from build123d import *

# Parameters (mm, degrees)
F1_DEPTH  = 5
F2_W      = 18
F2_H      = 15
F2_H_2    = 20
F3_DEPTH  = 20
F4_R      = 4
F5_DEPTH  = 25
F6_R      = 1.75
F6_R_2    = 11.25
F7_DEPTH  = 25
F8_W      = 42
F8_H      = 5
F9_DEPTH  = 20
F10_R     = 2.25
F11_DEPTH = 25
F12_DEPTH = 2
F13_R     = 4
F14_R     = 0.6


with BuildPart() as f1:
    # F0 (on Front) → F1 (new body)
    with BuildSketch(Plane.XZ):
        Polygon((-49.7673791122, 6.8827710084), (-49.7673791122, -8.1172289916), (28.2326208878, -8.1172289916), (28.2326208878, 11.8827710084), (10.2326208878, 11.8827710084), (10.2326208878, 46.8827710084), (-31.7673791122, 46.8827710084), (-31.7673791122, 6.8827710084), align=None)
    extrude(amount=F1_DEPTH)

    # F2 (on face) → F3 (join)
    with BuildSketch(Plane.XZ.offset(5)):
        with Locations((-40.7673791122, -0.6172289916)):
            Rectangle(F2_W, F2_H)
        with Locations((19.2326208878, 1.8827710084)):
            Rectangle(F2_W, F2_H_2)
    extrude(amount=F3_DEPTH)

    # F4 (on face) → F5 (cut)
    with BuildSketch(Plane(origin=(0, 0, -8.1172289916), x_dir=(1, 0, 0), z_dir=(0, 0, -1))):
        with Locations((-40.7673791122, 14)):
            Circle(F4_R)
        with Locations((19.2326208878, 14)):
            Circle(F4_R)
    extrude(amount=-F5_DEPTH, mode=Mode.SUBTRACT)

    # F6 (on face) → F7 (cut)
    with BuildSketch(Plane.XZ.offset(5)):
        with Locations((-26.2673791122, 41.3827710084)):
            Circle(F6_R)
        with Locations((-26.2673791122, 10.3827710084)):
            Circle(F6_R)
        with Locations((-10.7673791122, 25.8827710084)):
            Circle(F6_R_2)
        with Locations((4.7326208878, 41.3827710084)):
            Circle(F6_R)
        with Locations((4.7326208878, 10.3827710084)):
            Circle(F6_R)
    extrude(amount=-F7_DEPTH, mode=Mode.SUBTRACT)

    # F8 (on face) → F9 (join)
    with BuildSketch(Plane.XZ.offset(5)):
        with Locations((-10.7673791122, -5.6172289916)):
            Rectangle(F8_W, F8_H)
    extrude(amount=F9_DEPTH)

    # F10 (on face) → F11 (cut)
    with BuildSketch(Plane.XY.offset(-3.1172289916)):
        with Locations((-23.2673791122, -14)):
            Circle(F10_R)
        with Locations((1.7326208878, -14)):
            Circle(F10_R)
    extrude(amount=-F11_DEPTH, mode=Mode.SUBTRACT)

    # F10 (on face) → F12 (cut)
    with BuildSketch(Plane.XY.offset(-3.1172289916)):
        Polygon((-21.24665317, -17.5), (-19.2259272279, -14), (-21.24665317, -10.5), (-25.2881050544, -10.5), (-27.3088309965, -14), (-25.2881050544, -17.5), align=None)
        with Locations((-23.2673791122, -14)):
            Circle(F10_R, mode=Mode.SUBTRACT)
        Polygon((3.75334683, -17.5), (5.7740727721, -14), (3.75334683, -10.5), (-0.2881050544, -10.5), (-2.3088309965, -14), (-0.2881050544, -17.5), align=None)
        with Locations((1.7326208878, -14)):
            Circle(F10_R, mode=Mode.SUBTRACT)
    extrude(amount=-F12_DEPTH, mode=Mode.SUBTRACT)

    # F13
    f13_edges = [f1.edges().sort_by_distance(p)[0] for p in [
        (-49.767379, -25, -0.617229),
        (28.232621, -25, 1.882771),
        (28.232621, 0, 1.882771),
        (-49.767379, 0, -0.617229),
        (-31.767379, -2.5, 46.882771),
        (10.232621, -2.5, 46.882771),
        (-31.767379, -2.5, 6.882771),
        (10.232621, -2.5, 11.882771),
    ]]
    fillet(f13_edges, radius=F13_R)

    # F14
    f14_edges = [f1.edges().sort_by_distance(p)[0] for p in [
        (-22.017379, 0, 25.882771),
        (-22.017379, -5, 25.882771),
    ]]
    fillet(f14_edges, radius=F14_R)


solid = f1.part
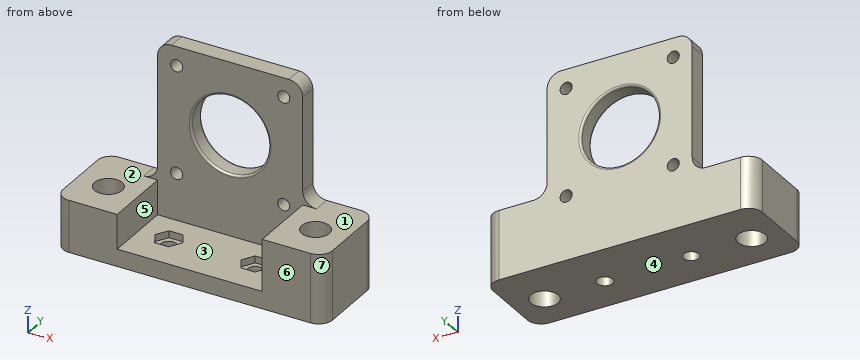
Build history of the part. All positions in model axes, mm. Face numbers are marked on the shaded views. A direction names the side the tool comes from. Coordinates: 2 decimals unless noted, no trailing zeros. Order: outer loops, then holes, each group sorted by start corner. A loop starts at its lowest first (then second) coordinate and runs counter-clockwise, first axis right, second up. Notation, with made-up numbers: M 65,55 L 124,55 A20 ccw 124,94 Z; hole C 40,-26.5 d4. An arc over 180 degrees is marked long. One line per question, with ' | ' between items. Start each with the question number.
Q1. Saw through at D-D (x = -30.5). List the corners of the cut face in (y, z), then the cut area to 3 significant figures.
Q2. Flat gauge pins, fed straight in: pin 1 Ø3 at (x, z) = (-17, 12.5) entering from -Y; pin 2 Ø3.5 at (x, y) = (-22, -13.5) entering from +Z; pin 3 Ø5.5 at (x, y) = (-37, -13.5) entering from +Z; pin 4 Ø7 at (x, y) = (19.23, -14) entering from -Z. Where does each tip first touch, or does it go through?
Q3. Saw through at C-C (y = -19). List the corners of the cut face in (x, z), then the cut area to 3 significant figures.
Q4. Probe L1, parallel to X at y = -14, z = 2.5; L2, parallel to X at y = -7, z = 0; L3, parallel to Z at x = 16, y = -23. List the from-to ranges inside material, lowest first. Write a range as from..to.
Q5. Saw through at B-B (x = -41.5). List the corners of the cut face in (y, z).
Q6. 3-axis set-ups, long thin cutter, end or side, ignore diameter. For the marked faces 1, 2, 3 and 4: which of +Z, -Z, +X, -X, +Y, -Y reach the whole face in a straight line?
Q7. Saw through at A-A (z = -2). List the corners of the cut face in (x, y), then the cut area to 3 significant figures.
Q8. Two-plate mould, pull along X, no slides. Class the marked faces 5, 6 and 7: +X half, -X half, draft (parallel to the pull), parting line (faces both ways), or undercut.
Check values:
1) outline: M -25,-8.12 L 0,-8.12 L 0,45.8 L -5,45.8 L -5,-3.12 L -25,-3.12 Z | area: 370 mm2
2) pin 1: stops at y = -5 | pin 2: stops at z = -5.12 | pin 3: stops at z = 6.88 | pin 4: passes through
3) outline: M -49.77,-8.12 L 28.23,-8.12 L 28.23,11.88 L 10.23,11.88 L 10.23,-3.12 L -31.77,-3.12 L -31.77,6.88 L -49.77,6.88 Z | area: 840 mm2
4) L1: x = -49.77..-44.77, -36.77..-31.77, 10.23..15.23, 23.23..28.23 | L2: x = -49.77..-31.77, 10.23..28.23 | L3: z = -8.12..11.88
5) outline: M -25,-8.12 L -17.93,-8.12 L -17.93,6.88 L -25,6.88 Z; M -10.07,-8.12 L 0,-8.12 L 0,6.88 L -10.07,6.88 Z
6) face 1: +Z, +X, -Y | face 2: +Z, -X, -Y | face 3: +Z, -Y | face 4: -Z, +X, -X, +Y, -Y
7) outline: M -49.77,-21 A4 ccw -45.77,-25 L -31.77,-25 L -31.77,-5 L 10.23,-5 L 10.23,-25 L 24.23,-25 A4 ccw 28.23,-21 L 28.23,-4 A4 ccw 24.23,0 L -45.77,0 A4 ccw -49.77,-4 Z; hole C -40.77,-14 d8; hole C 19.23,-14 d8 | area: 996 mm2
8) face 5: undercut | face 6: draft | face 7: +X half
